```python
from build123d import *

# Parameters (mm, degrees)
RESSALTO_EXTRUS_O1_DEPTH   = 25
ESBO_O5_W                  = 4.3
ESBO_O5_H                  = 15.6
ESBO_O5_W_2                = 26
ESBO_O5_H_2                = 14.2
CORTE_EXTRUS_O4_DEPTH      = 1
CORTE_EXTRUS_O4_DEPTH_BACK = 16
RESSALTO_EXTRUS_O2_DEPTH   = 2.5


with BuildPart() as part:
    # Esboço1 → Ressalto-extrusão1 (new body, symmetric)
    with BuildSketch(Plane.XY):
        Polygon((26, 0), (0, 0), (0, 15), (8, 15), (8, 13), (15.5, 5.5), (23, 13), (23, 15), (26, 15), align=None)
    extrude(amount=RESSALTO_EXTRUS_O1_DEPTH, both=True)

    # Esboço5 → Corte-extrusão4 (cut, two sides)
    with BuildSketch(Plane(origin=(0, 15, 0), x_dir=(1, 0, 0), z_dir=(0, 1, 0))) as corte_extrus_o4_sk:
        with Locations((5.85, 0)):
            Rectangle(ESBO_O5_W, ESBO_O5_H)
        with Locations((13, 17.9)):
            Rectangle(ESBO_O5_W_2, ESBO_O5_H_2)
        with Locations((13, -17.9)):
            Rectangle(ESBO_O5_W_2, ESBO_O5_H_2)
    extrude(amount=CORTE_EXTRUS_O4_DEPTH, mode=Mode.SUBTRACT)
    extrude(corte_extrus_o4_sk.sketch, amount=-CORTE_EXTRUS_O4_DEPTH_BACK, mode=Mode.SUBTRACT)

    # Esboço6 → Ressalto-extrusão2 (add, symmetric)
    with BuildSketch(Plane.XY):
        Polygon((0, 8.5), (-3, 4), (-3, 1), (-2, 1), (0, 4), align=None)
    extrude(amount=RESSALTO_EXTRUS_O2_DEPTH, both=True)


solid = part.part
```
The listing builds one solid part. Answer for the finished solid, in the listing's coordinates (mm). A direction names the side the tool comes from. Coordinates: 2 decimals unless noted, no trailing zeros. Write each loop counter-clockwise with the first axis right and the second up, starting at its lowest first coordinate (ties: lowest second). Pieces come first, ordered by that corner, then holes. Notation, with made-up numbers: (56, 11.25) - (73, 11.25) arc R12 cw to (73, 18.25) - close; hole circle Ø4 at (89.5, 70). An arc over 180 degrees is marked (long way). Return JSON: item names as keys, results as strings. Group by question number.
1. A cutting plane is placed at A-A, the plane y = 9. Determine the outline of the cut face in (x, z), plus the area to 3 significant figures.
2. A cutting plane is placed at C-C, the plane z = -0.25. Determine the outline of the cut face in (x, y).
3. Given pin 1 (1 mm diameter, centred on y = 6.5, z = 6.5, fed in from -X); pin 2 (1.5 mm diameter, centred on x = -1, y = 6.5, fed in from -Z); pin 3 (3 mm diameter, centred on x = 19, z = 7, fed in from +Y), each flat-ended and moving along its own axis, determine where each tip first touches the part or whether it passes through.
4. Determine the mould class of faces 4 (the flat face through (26, 8, 0)), 5 (the flat face through (16, 0, 0)), 6 (the flat face through (8, 14, 9)) for opening direction X: released by +X, released by -X, zero draft, split by the parting line, or undercut.
5. Which of the six approach directions +Z, -Z, +X, -X, +Y, -Y give full straight-line access (tool end or side, diameter ignored) to faces 1 (the flat face through (-2, 4, -2.5)), 2 (the flat face through (3.7, 8, 0)), 3 (the flat face through (8, 14, -9))?
6. A cutting plane is placed at D-D, the plane x = 7.25. Determine the outline of the cut face in (y, z).
7. Straight lines are drawn through the part: L1, parallel to Z at x = 6.25, y = 2.25; L2, parallel to X at y = 12, z = -5.5; L3, parallel to X at y = 3.25, z = -4. For each, find the intervals that lie inside material, in ascending order.
8. A cutting plane is placed at B-B, the plane y = 13.5. Determine the outline of the cut face in (x, z), plus the area to 3 significant figures.
Ans:
{
 "1": {"outline": "(0, -10.8) - (12, -10.8) - (12, 10.8) - (0, 10.8) - close; (19, -10.8) - (26, -10.8) - (26, 10.8) - (19, 10.8) - close; hole (3.7, -7.8) - (8, -7.8) - (8, 7.8) - (3.7, 7.8) - close", "area": "343 mm²"},
 "2": {"outline": "(-3, 1) - (-2, 1) - (0, 4) - (0, 0) - (3.7, 0) - (3.7, 15) - (0, 15) - (0, 8.5) - (-3, 4) - close; (8, 0) - (26, 0) - (26, 15) - (23, 15) - (23, 13) - (15.5, 5.5) - (8, 13) - close"},
 "3": {"pin 1": "x = 0", "pin 2": "z = -2.5", "pin 3": "y = 10.5"},
 "4": {"face 4": "released by +X", "face 5": "zero draft", "face 6": "undercut"},
 "5": {"face 1": "-Z, -X, +Y, -Y", "face 2": "+Y, -Y", "face 3": "+Z, -Z, +Y"},
 "6": {"outline": "(0, -10.8) - (15, -10.8) - (15, -7.8) - (0, -7.8) - close; (0, 7.8) - (15, 7.8) - (15, 10.8) - (0, 10.8) - close"},
 "7": {"L1": "-10.8 to -7.8, 7.8 to 10.8", "L2": "0 to 3.7, 8 to 9, 22 to 26", "L3": "0 to 3.7, 8 to 26"},
 "8": {"outline": "(0, -10.8) - (8, -10.8) - (8, -7.8) - (3.7, -7.8) - (3.7, 7.8) - (8, 7.8) - (8, 10.8) - (0, 10.8) - close; (23, -10.8) - (26, -10.8) - (26, 10.8) - (23, 10.8) - close", "area": "171 mm²"}
}
